Can you work these out from the drawing? Everything is in mm from the part's minimum corner. A direction names the side the tool comes from. Coordinates: 2 decimals unless noted, no trailing zeros. Loops run counter-clockwise (first coordinate to the right, second up) from the corner with the lowest first, then second, coordinate; pieces in that order, holes last. Notation, with made-up numbers: (77.25, 28.25) -> (113.25, 28.25) arc R31 cw to (113.25, 65.25) -> close; hole circle Ø9 at (-12, 23). An arc over 180 degrees is marked (long way). One line per question, with ' | ' between items.
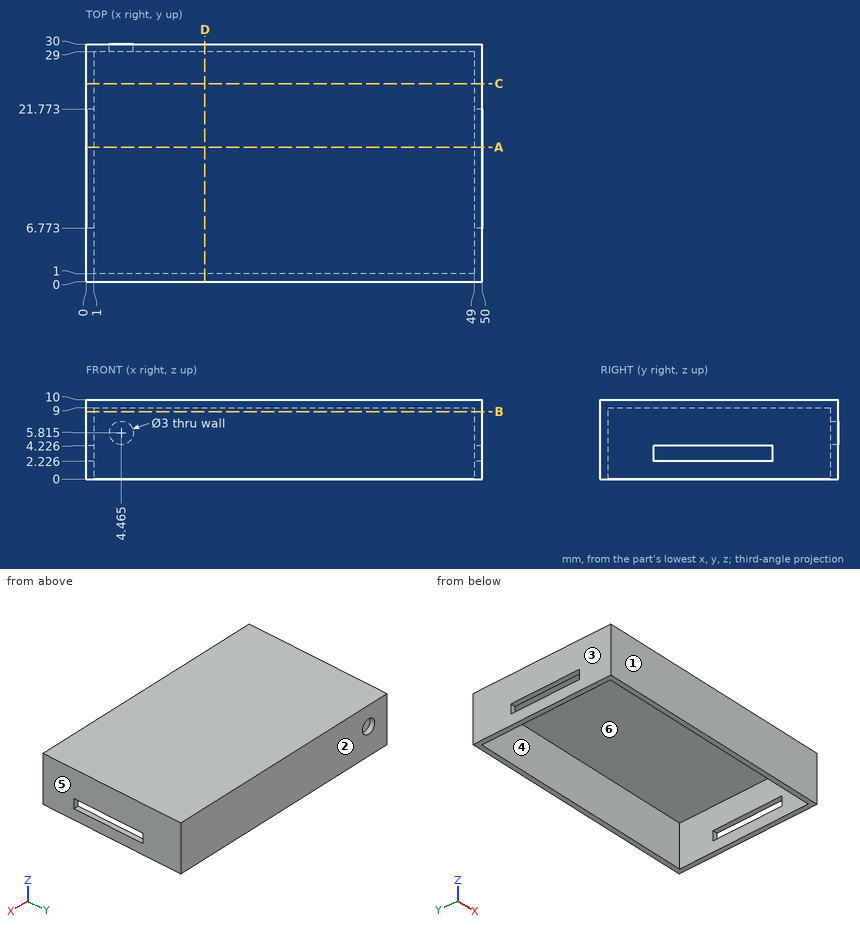
Q1. Imagine slicing it at D-D on x = 15. Write out the boundary of the cut face in (y, z).
Values follow:
outline: (0, 0) -> (1, 0) -> (1, 9) -> (29, 9) -> (29, 0) -> (30, 0) -> (30, 10) -> (0, 10) -> close
Q2. Imagine slicing it at C-C on y = 25. Write out the boundary of the cut face in (x, z).
Values follow:
outline: (0, 0) -> (1, 0) -> (1, 9) -> (49, 9) -> (49, 0) -> (50, 0) -> (50, 10) -> (0, 10) -> close
Q3. Please list where these lines run through material, in increasing order: L1, parallel to Y at x = 22, z = 1; L2, parallel to X at y = 22.5, z = 4.75; L3, parallel to Z at x = 6.5, y = 17.25. Write a range as [from, to].
Values follow:
L1: y = [0, 1], [29, 30] | L2: x = [0, 1], [49, 50] | L3: z = [9, 10]
Q4. Imagine slicing it at A-A on y = 17. Write out the boundary of the cut face in (x, z).
Values follow:
outline: (0, 0) -> (1, 0) -> (1, 2.23) -> (0, 2.23) -> close; (0, 4.23) -> (1, 4.23) -> (1, 9) -> (49, 9) -> (49, 4.23) -> (50, 4.23) -> (50, 10) -> (0, 10) -> close; (49, 0) -> (50, 0) -> (50, 2.23) -> (49, 2.23) -> close
Q5. We'd pull the mould along Y, two halves only. Please class the marked faces 1, 2, 3 and 4: released by +Y, released by -Y, zero draft, split by the parting line, or undercut.
Values follow:
face 1: released by -Y | face 2: released by +Y | face 3: zero draft | face 4: undercut
Q6. For the marked faces 5 and 6, which set-ups out of +Z, -Z, +X, -X, +Y, -Y let a thin tool reach every point of the face, with its end or its side?
Values follow:
face 5: +Z, -Z, +X, +Y, -Y | face 6: -Z
Q7. Imagine slicing it at B-B on z = 8.5. Write out the boundary of the cut face in (x, y).
Values follow:
outline: (0, 0) -> (50, 0) -> (50, 30) -> (0, 30) -> close; hole (1, 1) -> (49, 1) -> (49, 29) -> (1, 29) -> close
Q8. For pin 1 (1 mm diameter, centred on x = 28, y = 13.5, fed in from -Z), with a flat end and sliding along its axis, tell me the tip position at first contact or that it passes through.
Values follow:
pin 1: stops at z = 9
